```python
from build123d import *

# Parameters (mm, degrees)
SKETCH1_W           = 12.171
SKETCH1_H           = 11
BOSS_EXTRUDE1_DEPTH = 80
SKETCH2_R           = 1.5
CUT_EXTRUDE1_DEPTH  = 15
SKETCH4_R           = 1.5
CUT_EXTRUDE2_DEPTH  = 27


with BuildPart() as part:
    # Sketch1 → Boss-Extrude1 (new body)
    with BuildSketch(Plane.XY):
        with Locations((6.0855, 5.5)):
            Rectangle(SKETCH1_W, SKETCH1_H)
    extrude(amount=BOSS_EXTRUDE1_DEPTH)

    # Sketch2 → Cut-Extrude1 (cut)
    with BuildSketch(Plane(origin=(0, 11, 0), x_dir=(1, 0, 0), z_dir=(0, 1, 0))):
        with Locations((3.17, -61)):
            Circle(SKETCH2_R)
        with Locations((9.171, -61)):
            Circle(SKETCH2_R)
        with Locations((3.17, -19)):
            Circle(SKETCH2_R)
        with Locations((9.171, -19)):
            Circle(SKETCH2_R)
    extrude(amount=-CUT_EXTRUDE1_DEPTH, mode=Mode.SUBTRACT)

    # Sketch4 → Cut-Extrude2 (cut)
    with BuildSketch(Plane(origin=(0, 11, 0), x_dir=(1, 0, 0), z_dir=(0, 1, 0))):
        with Locations((6.085, -75)):
            Circle(SKETCH4_R)
        with Locations((6.085, -5)):
            Circle(SKETCH4_R)
    extrude(amount=-CUT_EXTRUDE2_DEPTH, mode=Mode.SUBTRACT)


solid = part.part
```
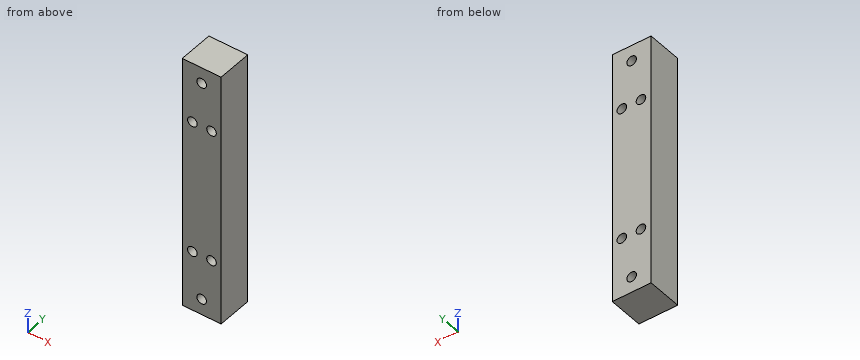
The listing builds one solid part. Answer for the finished solid, in the listing's coordinates (mm). Give positions to 0.01 mm unless a question says otherwise; leave off trailing zeros. Order: outer loops, then holes, each group sorted by start corner. A loop starts at its lowest first (then second) coordinate and runs counter-clockwise, first axis right, second up. Notation, with made-up numbers: (7.25, -34) - (20.25, -34) arc R25 cw to (20.25, -8) - close; hole circle Ø11 at (44.5, -18). An arc over 180 degrees is marked (long way). Use one line per item in the form item = value. Start each with the question number.
(1) A cutting plane is placed at D-D, the plane z = 75. Write down the section's boundary in (x, y) (3 decimals).
(2) Consider line 1 (X direction, y = 6, z = 61); line 2 (Z direction, x = 9, y = 6.5); line 3 (Z direction, x = 8, y = 8.5). Determine where each line is inside the solid, lowest interval first. Write a range as from..to.
(3) A flat-ended cylindrical pin translates along its axis: pin 1 Ø1.8 at (x, z) = (9.171, 61) entering from -Y. Find the tip coordinate at first contact, or state that the pin passes through.
(4) A cutting plane is placed at B-B, the plane x = 3.17. Write down the section's boundary in (y, z).
(5) A cutting plane is placed at C-C, the plane y = 8. Write down the section's boundary in (x, z) (3 decimals), then the cut area to 3 significant figures.
(6) A cutting plane is placed at A-A, the plane z = 19. Write down the section's boundary in (x, y), then the cut area to 3 significant figures.
Ans:
q1.outline = (0, 0) - (4.585, 0) - (4.585, 11) - (0, 11) - close; (7.585, 0) - (12.171, 0) - (12.171, 11) - (7.585, 11) - close
q2.line_1 = 0..1.67, 4.67..7.67, 10.67..12.17
q2.line_2 = 0..17.51, 20.49..59.51, 62.49..80
q2.line_3 = 0..18.06, 19.94..60.06, 61.94..80
q3.pin_1 = through
q4.outline = (0, 0) - (11, 0) - (11, 17.5) - (0, 17.5) - close; (0, 20.5) - (11, 20.5) - (11, 59.5) - (0, 59.5) - close; (0, 62.5) - (11, 62.5) - (11, 80) - (0, 80) - close
q5.outline = (0, 0) - (12.171, 0) - (12.171, 80) - (0, 80) - close; hole circle Ø3 at (3.17, 19); hole circle Ø3 at (3.17, 61); hole circle Ø3 at (6.085, 5); hole circle Ø3 at (6.085, 75); hole circle Ø3 at (9.171, 19); hole circle Ø3 at (9.171, 61)
q5.area = 931 mm^2
q6.outline = (0, 0) - (1.67, 0) - (1.67, 11) - (0, 11) - close; (4.67, 0) - (7.67, 0) - (7.67, 11) - (4.67, 11) - close; (10.67, 0) - (12.17, 0) - (12.17, 11) - (10.67, 11) - close
q6.area = 67.9 mm^2
